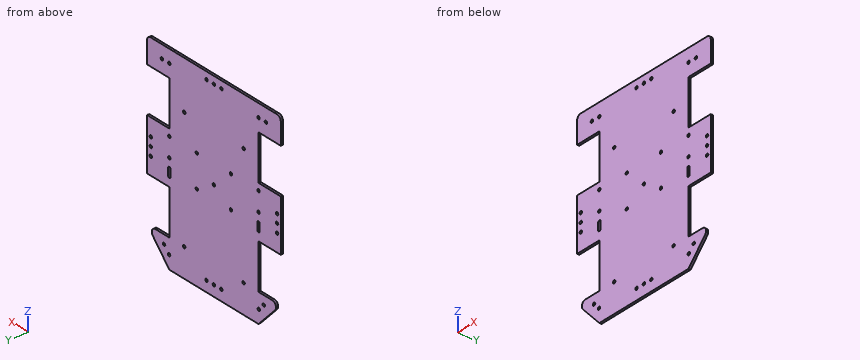
```python
from build123d import *

# Parameters (mm, degrees)
BOSS_EXTRUDE1_DEPTH = 2.5
FILLET1_R           = 5
FILLET2_R           = 5
SKETCH2_R           = 1.65
CUT_EXTRUDE1_DEPTH  = 232.152006264
SKETCH3_R           = 1.65
CUT_EXTRUDE2_DEPTH  = 10
SKETCH4_R           = 1.65
CUT_EXTRUDE3_DEPTH  = 10
SKETCH5_R           = 1.65
CUT_EXTRUDE4_DEPTH  = 10
SKETCH6_R           = 1.65
CUT_EXTRUDE5_DEPTH  = 10
SKETCH8_R           = 1.65
CUT_EXTRUDE6_DEPTH  = 10
SKETCH9_R           = 1.65
CUT_EXTRUDE7_DEPTH  = 10


with BuildPart() as part:
    # Sketch1 → Boss-Extrude1 (new body)
    with BuildSketch(Plane(origin=(0, 0, 0), x_dir=(1, 0, 0), z_dir=(0, 1, 0))):
        Polygon((0, 0), (0, 60), (30, 60), (30, 112), (0, 112), (30, 145), (150, 145), (180, 112), (150, 112), (150, 60), (180, 60), (180, 0), (150, 0), (150, -52), (180, -52), (180, -82), (0, -82), (0, -52), (30, -52), (30, 0), align=None)
    extrude(amount=BOSS_EXTRUDE1_DEPTH)

    # Fillet1
    fillet1_edges = [part.edges().sort_by_distance(p)[0] for p in [
        (180, 1.25, 82),
        (0, 1.25, 82),
    ]]
    fillet(fillet1_edges, radius=FILLET1_R)

    # Fillet2
    fillet2_edges = [part.edges().sort_by_distance(p)[0] for p in [
        (0, 1.25, -112),
        (180, 1.25, -112),
    ]]
    fillet(fillet2_edges, radius=FILLET2_R)

    # Sketch2 → Cut-Extrude1 (cut, through all)
    with BuildSketch(Plane(origin=(0, 2.5, 0), x_dir=(1, 0, 0), z_dir=(0, 1, 0))):
        with Locations(Location((30, 30, 0), (0, 0, 270))):
            Circle(SKETCH2_R)
        with Locations(Location((30, -67, 0), (0, 0, 270))):
            Circle(SKETCH2_R)
        with Locations(Location((50, 112, 0), (0, 0, 270))):
            Circle(SKETCH2_R)
        with Locations(Location((50, -26, 0), (0, 0, 270))):
            Circle(SKETCH2_R)
        with Locations(Location((150, -67, 0), (0, 0, 90))):
            Circle(SKETCH2_R)
        with Locations(Location((130, -26, 0), (0, 0, 90))):
            Circle(SKETCH2_R)
        with Locations(Location((150, 30, 0), (0, 0, 90))):
            Circle(SKETCH2_R)
        with Locations(Location((130, 112, 0), (0, 0, 90))):
            Circle(SKETCH2_R)
        with Locations(Location((20, -67, 0), (0, 0, 270))):
            Circle(SKETCH2_R)
        with Locations(Location((160, -67, 0), (0, 0, 90))):
            Circle(SKETCH2_R)
        with BuildLine():
            Line((28.35, 41), (28.35, 49))
            ThreePointArc((28.35, 49), (30, 50.65), (31.65, 49))
            Line((31.65, 49), (31.65, 41))
            ThreePointArc((31.65, 41), (30, 39.35), (28.35, 41))
        make_face()
        with BuildLine():
            Line((151.65, 41), (151.65, 49))
            ThreePointArc((151.65, 49), (150, 50.65), (148.35, 49))
            Line((148.35, 49), (148.35, 41))
            ThreePointArc((148.35, 41), (150, 39.35), (151.65, 41))
        make_face()
    extrude(amount=-CUT_EXTRUDE1_DEPTH, mode=Mode.SUBTRACT)

    # Sketch3 → Cut-Extrude2 (cut)
    with BuildSketch(Plane(origin=(0, 2.5, 0), x_dir=(1, 0, 0), z_dir=(0, 1, 0))):
        with Locations(Location((90, 132.681681985, 0), (0, 0, 270))):
            Circle(SKETCH3_R)
        with Locations(Location((80, 132.681681985, 0), (0, 0, 270))):
            Circle(SKETCH3_R)
        with Locations(Location((100, 132.681681985, 0), (0, 0, 90))):
            Circle(SKETCH3_R)
    extrude(amount=-CUT_EXTRUDE2_DEPTH, mode=Mode.SUBTRACT)

    # Sketch4 → Cut-Extrude3 (cut)
    with BuildSketch(Plane(origin=(0, 2.5, 0), x_dir=(1, 0, 0), z_dir=(0, 1, 0))):
        with Locations(Location((90, -73.500427327, 0), (0, 0, 270))):
            Circle(SKETCH4_R)
        with Locations(Location((80, -73.500427327, 0), (0, 0, 270))):
            Circle(SKETCH4_R)
        with Locations(Location((100, -73.500427327, 0), (0, 0, 90))):
            Circle(SKETCH4_R)
    extrude(amount=-CUT_EXTRUDE3_DEPTH, mode=Mode.SUBTRACT)

    # Sketch5 → Cut-Extrude4 (cut)
    with BuildSketch(Plane(origin=(0, 2.5, 0), x_dir=(1, 0, 0), z_dir=(0, 1, 0))):
        with Locations(Location((5, 30, 0), (0, 0, 270))):
            Circle(SKETCH5_R)
        with Locations(Location((5, 40, 0), (0, 0, 270))):
            Circle(SKETCH5_R)
        with Locations(Location((5, 20, 0), (0, 0, 270))):
            Circle(SKETCH5_R)
        with Locations(Location((175, 20, 0), (0, 0, 90))):
            Circle(SKETCH5_R)
        with Locations(Location((175, 30, 0), (0, 0, 90))):
            Circle(SKETCH5_R)
        with Locations(Location((175, 40, 0), (0, 0, 90))):
            Circle(SKETCH5_R)
    extrude(amount=-CUT_EXTRUDE4_DEPTH, mode=Mode.SUBTRACT)

    # Sketch6 → Cut-Extrude5 (cut)
    with BuildSketch(Plane(origin=(0, 2.5, 0), x_dir=(1, 0, 0), z_dir=(0, 1, 0))):
        with Locations(Location((90, 30, 0), (0, 0, 270))):
            Circle(SKETCH6_R)
    extrude(amount=-CUT_EXTRUDE5_DEPTH, mode=Mode.SUBTRACT)

    # Sketch8 → Cut-Extrude6 (cut)
    with BuildSketch(Plane(origin=(0, 2.5, 0), x_dir=(1, 0, 0), z_dir=(0, 1, 0))):
        with Locations(Location((29.564293781, 129.654654412, 0), (0, 0, 270))):
            Circle(SKETCH8_R)
        with Locations(Location((22.837565841, 122.255253678, 0), (0, 0, 270))):
            Circle(SKETCH8_R)
        with Locations(Location((157.162434159, 122.255253678, 0), (0, 0, 90))):
            Circle(SKETCH8_R)
        with Locations(Location((150.435706219, 129.654654412, 0), (0, 0, 90))):
            Circle(SKETCH8_R)
    extrude(amount=-CUT_EXTRUDE6_DEPTH, mode=Mode.SUBTRACT)

    # Sketch9 → Cut-Extrude7 (cut)
    with BuildSketch(Plane(origin=(0, 2.5, 0), x_dir=(1, 0, 0), z_dir=(0, 1, 0))):
        with Locations(Location((30, 7.996739715, 0), (0, 0, 270))):
            Circle(SKETCH9_R)
        with Locations(Location((67, 44.996739715, 0), (0, 0, 270))):
            Circle(SKETCH9_R)
        with Locations(Location((67, 7.996739715, 0), (0, 0, 270))):
            Circle(SKETCH9_R)
        with Locations(Location((150, 7.996739715, 0), (0, 0, 90))):
            Circle(SKETCH9_R)
        with Locations(Location((113, 7.996739715, 0), (0, 0, 90))):
            Circle(SKETCH9_R)
        with Locations(Location((113, 44.996739715, 0), (0, 0, 90))):
            Circle(SKETCH9_R)
    extrude(amount=-CUT_EXTRUDE7_DEPTH, mode=Mode.SUBTRACT)


solid = part.part
```
CAD build for the part. Positions are in the model's coordinates, mm. Coordinates: 2 decimals unless noted, no trailing zeros.
(1) Flat gauge pins, fed straight in: pin 1 (2 mm diameter, centred on x = 30, z = 67, fed in from -Y); pin 2 (1 mm diameter, centred on x = 26, y = 1.5, fed in from -Z). Where does each tip first touch, or does it go through?
(2) Cut at A-A, the plane y = 0.85. Count the separate pieces of the cut face and the enclosed holes in it, and give its area (3 significant figures).
(3) Drill centre lines: probe 1 along X at (y, z) = (1.1, -30); probe 2 along X at (y, z) = (0.8, -20); probe 3 along X at (y, z) = (0.8, 26). Where is each one in solid material? Low to high.
Geometry says:
1. pin 1: passes through
1. pin 2: stops at z = -141.15
2. separate pieces: 1
2. enclosed holes: 35
2. area: 33,200 mm2
3. probe 1: x = 0 to 3.35, 6.65 to 28.35, 31.65 to 88.35, 91.65 to 148.35, 151.65 to 173.35, 176.65 to 180
3. probe 2: x = 0 to 3.35, 6.65 to 173.35, 176.65 to 180
3. probe 3: x = 30 to 48.35, 51.65 to 128.35, 131.65 to 150
